The figure shows three views and two pictorial views of one solid part (mm, origin at its lowest corner). Answer the questions. Round coordinates to 2 decimals unless told otherwise and drop trailing zeros. Order: outer loops, then holes, each group sorted by start corner. A loop starts at its lowest first (then second) coordinate and runs counter-clockwise, first axis right, second up. Notation, with made-up numbers: M -17,33.25 L 35,33.25 A15 ccw 35,53.25 Z; hole C 42.25,20 d5. An arc over 180 degrees is marked long. Return JSON: item names as keys, results as strings.
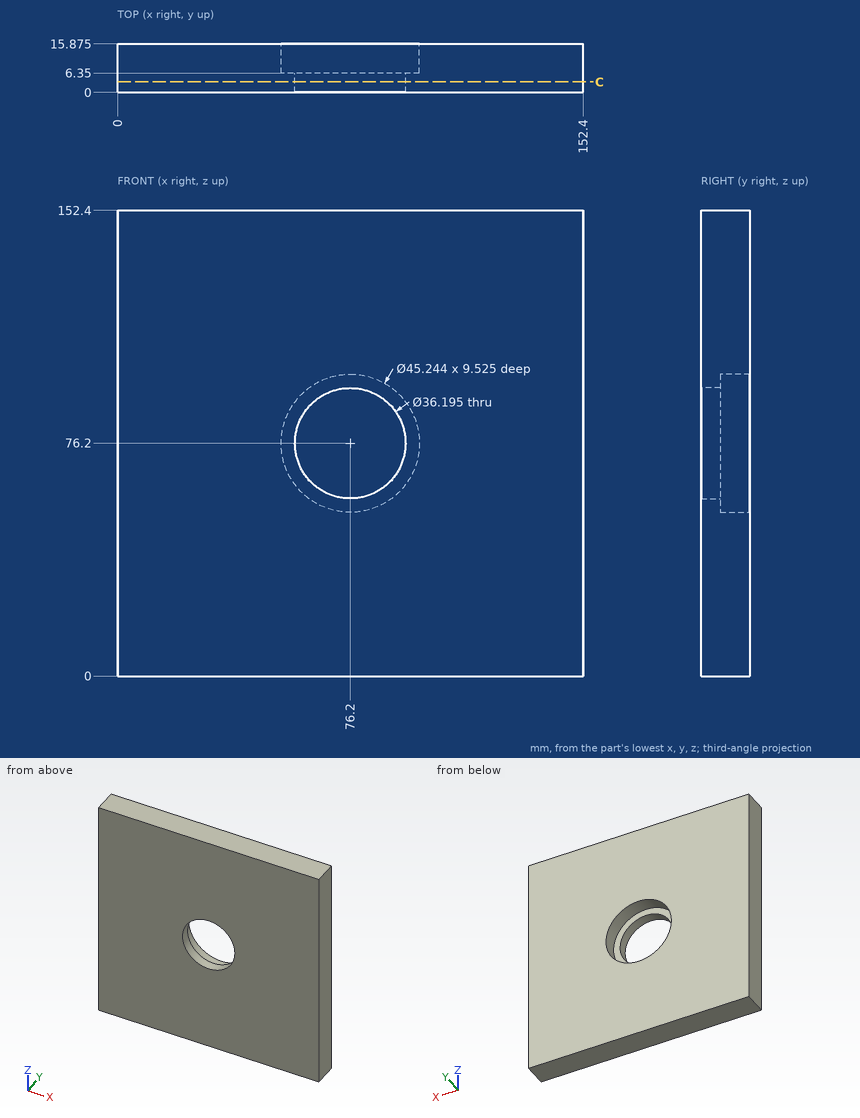
Item 1: This flat-tipped pin is pushed along its axis until it touches: pin 1 (22.5 mm diameter, centred on x = 86, z = 72.5, fed in from +Y). Where does it stop, or does it pass through?
Output:
{"pin 1": "stops at y = 6.35"}
Item 2: Consider line 1 along X through (y, z) = (8.5, 76.2); line 2 along Z through (x, y) = (67, 5.25) (1 decimal); line 3 along X through (y, z) = (2.75, 83). Determine where each line is inside the solid, lowest interval first. Write a range as [from, to].
Output:
{"line 1": "x = [0, 53.58], [98.82, 152.4]", "line 2": "z = [0, 60.6], [91.8, 152.4]", "line 3": "x = [0, 59.43], [92.97, 152.4]"}
Item 3: Find section C-C (y = 3.5). Determine the outline of the cut face in (x, z) (1 decimal).
Output:
{"outline": "M 0,0 L 152.4,0 L 152.4,152.4 L 0,152.4 Z; hole C 76.2,76.2 d36.2"}
